The listing builds one solid part. Answer for the finished solid, in the listing's coordinates (mm). Round coordinates to 2 decimals unless told otherwise and drop trailing zeros. Write each loop counter-clockwise with the first axis right and the second up, starting at its lowest first coordinate (ties: lowest second). Pieces come first, ordered by that corner, then holes.
(1) A cutting plane is placed at A-A, the plane z = 14.5. Give the vertices of the cut face in (x, y).
(2) A cutting plane is placed at B-B, the plane y = 6.5. Give the vertices of the cut face in (x, z).
(3) Each of these flat-tipped pins is pushed along its axis until it touches: pin 1 Ø2.5 at (y, z) = (5.71, 15.08) entering from -X; pin 2 Ø1 at (y, z) = (-11.5, 14) entering from -X. Where does it stop, or does it pass through?
(4) Find the intervals of material crossed by probe 1 along Y at (x, z) = (6, 14.75); probe 2 along Y at (x, z) = (4.5, 13.75); probe 3 along Z at (x, y) = (2.75, -20), in increasing order.
(5) A cutting plane is placed at C-C, the plane x = 4. Give the vertices of the cut face in (y, z) (1 decimal), and give its area (3 significant figures).
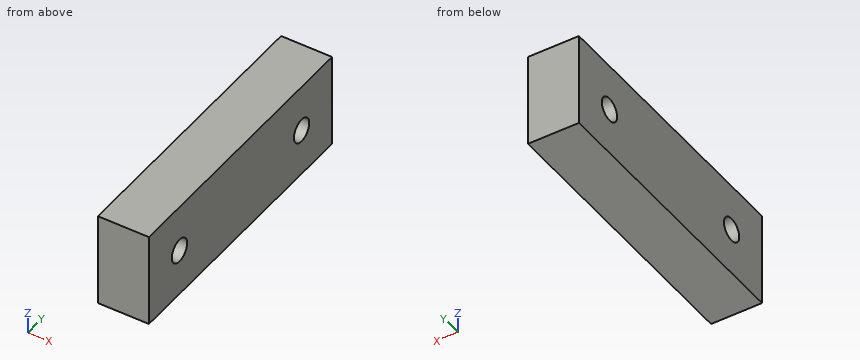
Autodesk Inventor part; units mm, degrees
ref_plane "YZ Plane" through (0, 0, 0) normal (1, 0, 0) x (0, 1, 0)
ref_plane "XZ Plane" through (0, 0, 0) normal (0, 1, 0) x (-1, 0, 0)
ref_plane "XY Plane" through (0, 0, 0) normal (0, 0, 1) x (1, 0, 0)
sketch "Sketch1" plane through (0, 0, 0) normal (1, 0, 0) x (0, 1, 0)
  line L0 (12.0622, 21.4347) -> (-26.0378, 21.4347)
  line L1 (-26.0378, 21.4347) -> (-26.0378, 8.7347)
  line L2 (-26.0378, 8.7347) -> (12.0622, 8.7347)
  line L3 (12.0622, 8.7347) -> (12.0622, 21.4347)
  point P0 (0, 0)
  dimension "d0" = 12.7
  dimension "d1" = 38.1
extrude "Extrusion1" add sketch "Sketch1" along normal blind 6.858
sketch "Sketch2" plane through (6.858, 0, 0) normal (1, 0, 0) x (0, 0, -1)
  line L0 (-8.7347, -26.0378) -> (-8.7347, 12.0622)
  line L1 (-8.7347, 12.0622) -> (-21.4347, 12.0622)
  point P0 (0, 0)
  point P1 (-15.0847, 5.7122)
  point P2 (-15.0847, -19.6878)
  dimension "d4" = 6.35
  dimension "d5" = 6.35
  dimension "d6" = 31.75
  dimension "d7" = 6.35
hole "Hole1" at (6.858, 5.7122, 15.0847) at (6.858, -19.6878, 15.0847) direction (-1, 0, 0) diameter 3.175 end through all
properties part number "GripperSliderBlock"
Solutions:
1. outline: (0, -26.04) - (6.86, -26.04) - (6.86, -21.16) - (0, -21.16) - close; (0, -18.21) - (6.86, -18.21) - (6.86, 4.24) - (0, 4.24) - close; (0, 7.19) - (6.86, 7.19) - (6.86, 12.06) - (0, 12.06) - close
2. outline: (0, 8.73) - (6.86, 8.73) - (6.86, 13.71) - (0, 13.71) - close; (0, 16.46) - (6.86, 16.46) - (6.86, 21.43) - (0, 21.43) - close
3. pin 1: passes through
3. pin 2: stops at x = 0
4. probe 1: y = -26.04 to -21.24, -18.14 to 4.16, 7.26 to 12.06
4. probe 2: y = -26.04 to -20.55, -18.83 to 4.85, 6.57 to 12.06
4. probe 3: z = 8.73 to 13.53, 16.64 to 21.43
5. outline: (-26, 8.7) - (12.1, 8.7) - (12.1, 21.4) - (-26, 21.4) - close; hole circle Ø3.2 at (-19.7, 15.1); hole circle Ø3.2 at (5.7, 15.1)
5. area: 468 mm2
